```python
from build123d import *

# Parameters (mm, degrees)
MAIN_EXTRUDE_DEPTH = 40
FILLET1_R          = 1
FILLET2_R          = 1
FILLET3_R          = 1
CUT_EXTRUDE1_DEPTH = 20


with BuildPart() as part:
    # Sketch1 → Main-Extrude (new body)
    with BuildSketch(Plane(origin=(0, 0, 0), x_dir=(1, 0, 0), z_dir=(0, 1, 0))):
        with BuildLine():
            Line((6.5, 11.159541063), (6.5, 7.659541063))
            ThreePointArc((6.5, 7.659541063), (6.80229201, 7.200289987), (7.343646203, 7.296350635))
            Line((7.343646203, 7.296350635), (11.187292407, 10.933160207))
            ThreePointArc((11.187292407, 10.933160207), (11.418502152, 11.264125084), (11.5, 11.659541063))
            Line((11.5, 11.659541063), (11.5, 16.659541063))
            ThreePointArc((11.5, 16.659541063), (11.418502152, 17.054957042), (11.187292407, 17.385921919))
            Line((11.187292407, 17.385921919), (7.343646203, 21.022731491))
            ThreePointArc((7.343646203, 21.022731491), (6.80229201, 21.118792139), (6.5, 20.659541063))
            Line((6.5, 20.659541063), (6.5, 17.159541063))
            Line((6.5, 17.159541063), (3, 17.159541063))
            Line((3, 17.159541063), (3, 26.109541063))
            Line((3, 26.109541063), (-1, 26.109541063))
            Line((-1, 26.109541063), (-1, 0.659541063))
            Line((-1, 0.659541063), (-19, 0.659541063))
            Line((-19, 0.659541063), (-19, -3.340458937))
            Line((-19, -3.340458937), (-4.999912017, -3.340458937))
            Line((-4.999912017, -3.340458937), (28.4, -3.340458937))
            Line((28.4, -3.340458937), (28.4, 0.659541063))
            Line((28.4, 0.659541063), (3, 0.659541063))
            Line((3, 0.659541063), (3, 11.159541063))
            Line((3, 11.159541063), (6.5, 11.159541063))
        make_face()
    extrude(amount=MAIN_EXTRUDE_DEPTH)

    # Fillet1
    fillet1_edges = [part.edges().sort_by_distance(p)[0] for p in [
        (28.4, 20, 3.340458937),
        (-19, 20, 3.340458937),
        (28.4, 20, -0.659541063),
    ]]
    fillet(fillet1_edges, radius=FILLET1_R)

    # Fillet2
    fillet2_edges = [part.edges().sort_by_distance(p)[0] for p in [
        (-19, 20, -0.659541063),
    ]]
    fillet(fillet2_edges, radius=FILLET2_R)

    # Fillet3
    fillet3_edges = [part.edges().sort_by_distance(p)[0] for p in [
        (-1, 20, -0.659541063),
    ]]
    fillet(fillet3_edges, radius=FILLET3_R)

    # Sketch5 → Cut-Extrude1 (cut)
    with BuildSketch(Plane.XZ):
        Polygon((-19, -0.659541063), (-4.518354444, -0.659541063), (-4.518354444, -5.516455238), (-1, -5.516455238), (-1, -0.659541063), (3, -0.659541063), (3, -5.516455238), (6.594635696, -5.516455238), (6.594635696, -0.659541063), (28.4, -0.659541063), (28.4, 3.340458937), (-19, 3.340458937), align=None)
    extrude(amount=-CUT_EXTRUDE1_DEPTH, mode=Mode.SUBTRACT)


solid = part.part
```
The listing builds one solid part. Answer for the finished solid, in the listing's coordinates (mm). A direction names the side the tool comes from. Round coordinates to 2 decimals unless told otherwise and drop trailing zeros. Order: outer loops, then holes, each group sorted by start corner. A loop starts at its lowest first (then second) coordinate and runs counter-clockwise, first axis right, second up. Notation, with made-up numbers: (80, 29) -> (130, 29) arc R35 ccw to (130, 65) -> close; hole circle Ø1 at (-2, -15). An arc over 180 degrees is marked (long way). Answer as CSV lines item,"result". Start each with the question number.
(1) The part is cut by section C-C (z = -2.5). Determine the outline of the cut face in (x, y), then the cut area to 3 significant figures.
(2) Flat-ended cylindrical pins translate along their axes: pin 1 Ø3 at (x, y) = (1.5, 9.5) entering from +Z; pin 2 Ø8.5 at (y, z) = (18, -7) entering from +X; pin 3 Ø10 at (x, y) = (19.5, 28.5) entering from -Z. Find the tip coordinate at first contact, or state that the pin passes through.
(3) Find the intervals of material crossed by probe 1 along X at (y, z) = (22, -8.5); probe 2 along X at (y, z) = (4, -21.25); probe 3 along Z at (x, y) = (-3, 33.5), in increasing order. Write a range as from..to.
(4) A tool of negligible diameter and unlimited length cuts with its end or side. For faces 1 (the face through (-10, 30, -0.66)), 2 (the face through (1, 10, -0.66)), 3 (the face through (6.5, 20, -19)), 4 (the face through (3, 20, -6)), 5 (the face through (15, 30, -0.66)), from which of +Z, -Z, +X, -X, +Y, -Y can it reach the whole face along a straight path? Write none if from no direction.
(5) The part is cut by section A-A (x = 5). Determine the outline of the cut face in (y, z), then the cut area to 3 significant figures.
(6) For a pull along X with two mould halves and no side action, classify faces 6 (the face through (5, 20, -11.16)), 7 (the face through (1, 20, -26.11)), 8 (the face through (-19, 30, 1)) as +X half, -X half, draft (parallel to the pull), parting line (faces both ways), or undercut.
(7) The part is cut by section B-B (y = 15). Determine the outline of the cut face in (x, z).
(8) The part is cut by section D-D (x = -13). Determine the outline of the cut face in (y, z), then the cut area to 3 significant figures.
Evaluation:
1,outline,"(-1, 0) -> (3, 0) -> (3, 40) -> (-1, 40) -> close"
1,area,"160 mm²"
2,pin 1,"z = -0.66"
2,pin 2,"x = 11.41"
2,pin 3,"z = -0.66"
3,probe 1,"-1..3, 6.5..8.62"
3,probe 2,"-1..3"
3,probe 3,"-0.66..3.34"
4,face 1,"-Z, -X, +Y, -Y"
4,face 2,"+Z, +X, -X, -Y"
4,face 3,"-Z, +Y, -Y"
4,face 4,"+Y, -Y"
4,face 5,"+X, +Y, -Y"
5,outline,"(0, -17.16) -> (40, -17.16) -> (40, -11.16) -> (0, -11.16) -> close; (20, -0.66) -> (40, -0.66) -> (40, 3.34) -> (20, 3.34) -> close"
5,area,"320 mm²"
6,face 6,"undercut"
6,face 7,"draft"
6,face 8,"-X half"
7,outline,"(-1, -26.11) -> (3, -26.11) -> (3, -17.16) -> (6.5, -17.16) -> (6.5, -20.66) arc R0.5 ccw to (7.34, -21.02) -> (11.19, -17.39) arc R1 ccw to (11.5, -16.66) -> (11.5, -11.66) arc R1 ccw to (11.19, -10.93) -> (7.34, -7.3) arc R0.5 ccw to (6.5, -7.66) -> (6.5, -11.16) -> (3, -11.16) -> (3, -0.66) -> (-1, -0.66) -> close"
8,outline,"(20, -0.66) -> (40, -0.66) -> (40, 3.34) -> (20, 3.34) -> close"
8,area,"80.0 mm²"
